from build123d import *

# Parameters (mm, degrees)
SKICA1_W                 = 50.278910674
SKICA1_H                 = 21.7
SKICA1_R                 = 1.6
P_IDAT_VYSUNUT_M1_DEPTH  = 8
SKICA2_R                 = 2.5
ODEBRAT_VYSUNUT_M1_DEPTH = 4
SKICA4_W                 = 12.327690559
SKICA4_H                 = 21.7
P_IDAT_VYSUNUT_M2_DEPTH  = 15
SKICA6_R                 = 5.406276896
P_IDAT_VYSUNUT_M3_DEPTH  = 21.7
SKICA7_R                 = 1.5
ODEBRAT_VYSUNUT_M3_DEPTH = 21.7
SKICA8_W                 = 8
SKICA8_H                 = 21.7
P_IDAT_VYSUNUT_M4_DEPTH  = 15
SKICA9_R                 = 1.6
ODEBRAT_VYSUNUT_M4_DEPTH = 15
SKICA10_R                = 11
P_IDAT_VYSUNUT_M5_DEPTH  = 7
ZKOSEN_1_SIZE            = 10
SKICA11_W                = 20.957821349
SKICA11_H                = 4.85
P_IDAT_VYSUNUT_M6_DEPTH  = 5


with BuildPart() as part:
    # Skica1 → Přidat vysunutím1 (new body)
    with BuildSketch(Plane.XY):
        with Locations((-8.927473885, -9.09140889)):
            Rectangle(SKICA1_W, SKICA1_H)
        with Locations((13.311981452, -16.59140889)):
            Circle(SKICA1_R, mode=Mode.SUBTRACT)
        with Locations((-6.688018548, -16.59140889)):
            Circle(SKICA1_R, mode=Mode.SUBTRACT)
        with Locations((-6.688018548, -1.59140889)):
            Circle(SKICA1_R, mode=Mode.SUBTRACT)
        with Locations((13.311981452, -1.59140889)):
            Circle(SKICA1_R, mode=Mode.SUBTRACT)
    extrude(amount=P_IDAT_VYSUNUT_M1_DEPTH)

    # Skica2 → Odebrat vysunutím1 (cut)
    with BuildSketch(Plane.XY.offset(8)):
        with Locations((13.311981452, -16.59140889)):
            Circle(SKICA2_R)
        with Locations((-6.688018548, -16.59140889)):
            Circle(SKICA2_R)
        with Locations((-6.688018548, -1.59140889)):
            Circle(SKICA2_R)
        with Locations((13.311981452, -1.59140889)):
            Circle(SKICA2_R)
    extrude(amount=-ODEBRAT_VYSUNUT_M1_DEPTH, mode=Mode.SUBTRACT)

    # Skica4 → Přidat vysunutím2 (add)
    with BuildSketch(Plane(origin=(0, 0, 0), x_dir=(-1, 0, 0), z_dir=(0, 0, -1))):
        with Locations((16.351863828, -9.09140889)):
            Rectangle(SKICA4_W, SKICA4_H)
    extrude(amount=P_IDAT_VYSUNUT_M2_DEPTH)

    # Skica6 → Přidat vysunutím3 (add)
    with BuildSketch(Plane(origin=(0, 1.75859111, 0), x_dir=(1, 0, 0), z_dir=(0, 1, 0))):
        Polygon((-22.515709107, 15), (-10.188018548, 15), (-7.585826442, 20.254970434), (20.97371307, 20.254970434), (20.97371307, 45.15), (4.741864117, 45.15), (-7.585826442, 45.15), align=None)
        with Locations(Location((8.208247023, 34.15, 0), (0, 0, 270))):
            Circle(SKICA6_R, mode=Mode.SUBTRACT)
    extrude(amount=-P_IDAT_VYSUNUT_M3_DEPTH)

    # Skica7 → Odebrat vysunutím3 (cut)
    with BuildSketch(Plane.XZ.offset(19.94140889)):
        with Locations(Location((2.551392773, -28.493145751, 0), (0, 0, 270))):
            Circle(SKICA7_R)
        with Locations(Location((13.865101272, -39.806854249, 0), (0, 0, 270))):
            Circle(SKICA7_R)
    extrude(amount=-ODEBRAT_VYSUNUT_M3_DEPTH, mode=Mode.SUBTRACT)

    # Skica8 → Přidat vysunutím4 (add)
    with BuildSketch(Plane.ZY.offset(34.066929222)):
        with Locations((4, -9.09140889)):
            Rectangle(SKICA8_W, SKICA8_H)
    extrude(amount=P_IDAT_VYSUNUT_M4_DEPTH)

    # Skica9 → Odebrat vysunutím4 (cut)
    with BuildSketch(Plane.XY.offset(8)):
        with Locations((-43.109107873, -9.09140889)):
            Circle(SKICA9_R)
    extrude(amount=-ODEBRAT_VYSUNUT_M4_DEPTH, mode=Mode.SUBTRACT)

    # Skica10 → Přidat vysunutím5 (add)
    with BuildSketch(Plane(origin=(20.97371307, 0, 0), x_dir=(0, 0, -1), z_dir=(1, 0, 0))):
        Polygon((8.074184901, 14.340387575), (20.254970434, 1.75859111), (20.254970434, -19.94140889), (45.15, -19.94140889), (45.15, 48.622184041), (8.074184901, 48.622184041), align=None)
        with Locations((24.65, 27.25859111)):
            Circle(SKICA10_R, mode=Mode.SUBTRACT)
    extrude(amount=P_IDAT_VYSUNUT_M5_DEPTH)

    # Zkosení1
    zkosen_1_edges = [part.edges().sort_by_distance(p)[0] for p in [
        (24.47371307, 48.622184041, -45.15),
        (24.47371307, 48.622184041, -8.074184901),
    ]]
    chamfer(zkosen_1_edges, length=ZKOSEN_1_SIZE)

    # Skica11 → Přidat vysunutím6 (add)
    with BuildSketch(Plane.XY.offset(8)):
        with Locations((-38.588018548, -0.66640889)):
            Rectangle(SKICA11_W, SKICA11_H)
        with Locations((-38.588018548, -17.51640889)):
            Rectangle(SKICA11_W, SKICA11_H)
    extrude(amount=P_IDAT_VYSUNUT_M6_DEPTH)


solid = part.part
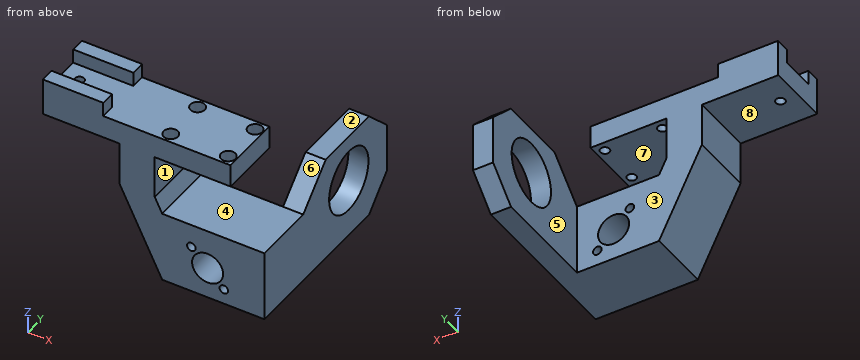
Could you check a few things on this model? Use its own coordinates, in mm. Face numbers are marked on the shaded views. A direction names the side the tool comes from. Coordinates: 2 decimals unless noted, no trailing zeros. Write each loop counter-clockwise with the first axis right and the second up, starting at its lowest first coordinate (ties: lowest second). Pieces come first, ordered by that corner, then holes. Notation, with made-up numbers: M 26,29.5 L 30,29.5 A34 ccw 30,59.5 Z; hole C 13.5,38.5 d1. An arc over 180 degrees is marked long. One line per question, with ' | ' between items.
1) Imagine slicing it at B-B, the plane y = 20. Write out the boundary of the cut face in (x, z).
Checks:
outline: M 20.97,-45.15 L 27.97,-45.15 L 27.97,-32.92 L 20.97,-32.92 Z; M 20.97,-16.38 L 27.97,-16.38 L 27.97,-8.07 L 20.97,-8.07 Z
2) If we mould it in two halves opening along Z, with no side actions, what happens to the marked faces 1, 2 and 3? For each: released by +Z, released by -Z, zero draft, split by the parting line, or undercut.
Checks:
face 1: undercut | face 2: released by +Z | face 3: zero draft
3) Imagine slicing it at D-D, the plane x = -25.5. Write out the boundary of the cut face in (y, z).
Checks:
outline: M -19.94,0 L 1.76,0 L 1.76,8 L -19.94,8 Z
4) For the marked faces 4, 5, 6, 7 and 8, which set-ups out of +Z, -Z, +X, -X, +Y, -Y let a thin tool reach every point of the face, with its end or its side?
Checks:
face 4: +X, -Y | face 5: +Z, -Z, -X, +Y | face 6: +Z, +X, -X, -Y | face 7: +X, +Y, -Y | face 8: -Z, -X, +Y, -Y
5) Imagine slicing it at A-A, the plane z = -10. Write out the boundary of the cut face in (x, y), and give its area (3 significant figures).
Checks:
outline: M -22.52,-19.94 L -10.19,-19.94 L -10.19,1.76 L -22.52,1.76 Z; M 20.97,12.35 L 27.97,12.35 L 27.97,40.55 L 20.97,40.55 Z | area: 465 mm²
6) For pin 1 Ø5.5 at (x, y) = (13.5, -16.5) entering from +Z; pin 2 Ø1.5 at (x, z) = (-40, 11) entering from +Y; pin 3 Ø4.5 at (y, z) = (-10, -4) entering from +X; pin 4 Ø4 at (x, y) = (-36.5, 2) entering from +Z, each with a flat end and sliding along its axis, tell me the tip position at first contact or that it passes through.
Checks:
pin 1: z = 8 | pin 2: y = 1.76 | pin 3: x = -10.19 | pin 4: z = 13
7) I need wall thicknesses on probe 1 along Y at (x, z) = (23, -24.65); probe 2 along Z at (x, y) = (-1, -11); probe 3 along Y at (x, z) = (5, -43). Which ranges of each line are inside material? Lowest first, please. Write a range as [from, to].
Checks:
probe 1: [-19.94, 16.26], [38.26, 48.62] | probe 2: [-45.15, -20.25], [0, 8] | probe 3: [-19.94, 1.76]
8) Imagine slicing it at C-C, the plane z = -34. Write out the boundary of the cut face in (x, y).
Checks:
outline: M -13.11,-19.94 L 2.8,-19.94 L 2.8,1.76 L -13.11,1.76 Z; M 13.61,-19.94 L 27.97,-19.94 L 27.97,21.46 L 20.97,21.46 L 20.97,1.76 L 13.61,1.76 Z; M 20.97,33.05 L 27.97,33.05 L 27.97,48.62 L 20.97,48.62 Z
